The listing builds one solid part. Answer for the finished solid, in the listing's coordinates (mm). Give positions to 0.01 mm unless a question says otherwise; leave off trailing zeros. Loops run counter-clockwise (first coordinate to the right, second up) from the corner with the lowest first, then second, coordinate; pieces in that order, holes last. Notation, with made-up numbers: (44.25, 74.5) - (63.25, 74.5) arc R10 ccw to (63.25, 79.5) - close; hole circle Ø8 at (89.25, 72.25). An arc over 180 degrees is marked (long way). Answer in a Markdown table with one row per item. Add a question column.
```python
from build123d import *

# Parameters (mm, degrees)
ESQUISSE1_R             = 15
BOSS_EXTRU_1_DEPTH      = 5
ESQUISSE2_R             = 2.95
ENL_V_MAT_EXTRU_1_DEPTH = 22.794494718
D_GAGEMENT_M2_51_D      = 2.7


with BuildPart() as part:
    # Esquisse1 → Boss.-Extru.1 (new body)
    with BuildSketch(Plane(origin=(0, 0, 0), x_dir=(1, 0, 0), z_dir=(0, 1, 0))):
        with Locations(Location((0, 0, 0), (0, 0, 270))):
            Circle(ESQUISSE1_R)
    extrude(amount=BOSS_EXTRU_1_DEPTH)

    # Esquisse2 → Enlèv. mat.-Extru.1 (cut, through all)
    with BuildSketch(Plane(origin=(0, 5, 0), x_dir=(1, 0, 0), z_dir=(0, 1, 0))):
        with Locations(Location((0, 0, 0), (0, 0, 270))):
            Circle(ESQUISSE2_R)
    extrude(amount=-ENL_V_MAT_EXTRU_1_DEPTH, mode=Mode.SUBTRACT)

    # Dégagement M2.51 (through all)
    with Locations(Plane(origin=(0, 5, 0), x_dir=(1, 0, 0), z_dir=(0, 1, 0))):
        with Locations((0, 0), (-12, 0), (-8.485281374, 8.485281374), (0, 12), (8.485281374, 8.485281374), (12, 0), (8.485281374, -8.485281374), (0, -12), (-8.485281374, -8.485281374)):
            Hole(D_GAGEMENT_M2_51_D / 2)


solid = part.part
```
(1) Find the intervals of material crossed by line 1 along Z through (x, y) = (0.5, 2.05); line 2 along Z through (x, y) = (9.5, 1.75); line 3 along X through (y, z) = (0.4, -9), in increasing order. Write a range as [from, to].
(2) The mould has two halves that part along Z. Classify faces 1 (the face through (-2.88, 2.54, -0.64)), 2 (the face through (0.2, 0, 3.1)), 3 (the face through (0.66, 2.465, -14.985)): pulls with the +Z half, pulls with the -Z half, needs draft (parallel to the pull), parting line crosses it, or undercut.
(3) A cutting plane is placed at D-D on z = 0. Determine the outline of the cut face in (x, y), plus the area to 3 significant figures.
(4) A cutting plane is placed at B-B on x = 12. Determine the outline of the cut face in (y, z).
(5) A cutting plane is placed at C-C on y = 1.6. Give the number of separate pieces and of enclosed holes in the cut face, plus the area to 3 significant figures.
(6) A cutting plane is placed at A-A on z = 12. Determine the outline of the cut face in (x, y), plus the area to 3 significant figures.
(7) Given pin 1 Ø1.6 at (x, z) = (8.49, -8.49) entering from +Y, flat-ended and moving along its own axis, determine where the tip first touches the part or whether it passes through.
Evaluation:
| question | item | result |
|---|---|---|
| 1 | line 1 | z = [-14.99, -13.25], [-10.75, -2.91], [2.91, 10.75], [13.25, 14.99] |
| 1 | line 2 | z = [-11.61, -9.38], [-7.59, 7.59], [9.38, 11.61] |
| 1 | line 3 | x = [-12, -9.73], [-7.24, 7.24], [9.73, 12] |
| 2 | face 1 | undercut |
| 2 | face 2 | needs draft |
| 2 | face 3 | parting line crosses it |
| 3 | outline | (-15, 0) - (-13.35, 0) - (-13.35, 5) - (-15, 5) - close; (-10.65, 0) - (-2.95, 0) - (-2.95, 5) - (-10.65, 5) - close; (2.95, 0) - (10.65, 0) - (10.65, 5) - (2.95, 5) - close; (13.35, 0) - (15, 0) - (15, 5) - (13.35, 5) - close |
| 3 | area | 93.5 mm² |
| 4 | outline | (0, -9) - (5, -9) - (5, -1.35) - (0, -1.35) - close; (0, 1.35) - (5, 1.35) - (5, 9) - (0, 9) - close |
| 5 | separate pieces | 1 |
| 5 | enclosed holes | 9 |
| 5 | area | 634 mm² |
| 6 | outline | (-9, 0) - (-1.35, 0) - (-1.35, 5) - (-9, 5) - close; (1.35, 0) - (9, 0) - (9, 5) - (1.35, 5) - close |
| 6 | area | 76.5 mm² |
| 7 | pin 1 | passes through |
